```python
from build123d import *

# Parameters (mm, degrees)
BOSS_EXTRUDE1_DEPTH = 5
SKETCH2_W           = 20.5
SKETCH2_H           = 30
SKETCH2_R           = 3
SKETCH2_R_2         = 1.5
BOSS_EXTRUDE2_DEPTH = 5
FILLET1_R           = 10.25


with BuildPart() as part:
    # Sketch1 → Boss-Extrude1 (new body)
    with BuildSketch(Plane(origin=(0, 0, 0), x_dir=(1, 0, 0), z_dir=(0, 1, 0))):
        Polygon((44.375484097, 7.788988346), (75.375484097, 7.788988346), (80.375484097, 7.788988346), (80.375484097, 12.788988346), (75.375484097, 12.788988346), (75.375484097, 18.288988346), (73.375484097, 18.288988346), (73.375484097, 17.188988346), (71.075484097, 17.188988346), (71.075484097, 18.288988346), (68.375484097, 18.288988346), (68.375484097, 21.288988346), (71.075484097, 21.288988346), (71.075484097, 22.388988346), (73.375484097, 22.388988346), (73.375484097, 21.288988346), (75.375484097, 21.288988346), (75.375484097, 26.788988346), (80.375484097, 26.788988346), (80.375484097, 31.788988346), (75.375484097, 31.788988346), (44.375484097, 31.788988346), (39.375484097, 31.788988346), (39.375484097, 26.788988346), (44.375484097, 26.788988346), (44.375484097, 21.288988346), (46.375484097, 21.288988346), (46.375484097, 22.388988346), (48.675484097, 22.388988346), (48.675484097, 21.288988346), (51.375484097, 21.288988346), (51.375484097, 18.288988346), (48.675484097, 18.288988346), (48.675484097, 17.188988346), (46.375484097, 17.188988346), (46.375484097, 18.288988346), (44.375484097, 18.288988346), (44.375484097, 12.788988346), (39.375484097, 12.788988346), (39.375484097, 7.788988346), align=None)
    extrude(amount=BOSS_EXTRUDE1_DEPTH)

    # Sketch2 → Boss-Extrude2 (add)
    with BuildSketch(Plane(origin=(0, 5, 0), x_dir=(1, 0, 0), z_dir=(0, 1, 0))):
        with Locations((59.875484097, -7.211011654)):
            Rectangle(SKETCH2_W, SKETCH2_H)
        with Locations(Location((59.875484097, -11.961011654, 0), (0, 0, 270))):
            Circle(SKETCH2_R, mode=Mode.SUBTRACT)
        with Locations(Location((59.875484097, -19.461011654, 0), (0, 0, 270))):
            Circle(SKETCH2_R_2, mode=Mode.SUBTRACT)
        with Locations(Location((52.375484097, -11.961011654, 0), (0, 0, 90))):
            Circle(SKETCH2_R_2, mode=Mode.SUBTRACT)
        with Locations(Location((67.375484097, -11.961011654, 0), (0, 0, 90))):
            Circle(SKETCH2_R_2, mode=Mode.SUBTRACT)
        with Locations(Location((59.875484097, -4.461011654, 0), (0, 0, 270))):
            Circle(SKETCH2_R_2, mode=Mode.SUBTRACT)
    extrude(amount=-BOSS_EXTRUDE2_DEPTH)

    # Fillet1
    fillet1_edges = [part.edges().sort_by_distance(p)[0] for p in [
        (49.625484097, 2.5, 22.211011654),
        (70.125484097, 2.5, 22.211011654),
    ]]
    fillet(fillet1_edges, radius=FILLET1_R - 0.0001)  # a hair under: the kernel refuses the full size


solid = part.part
```
CAD build for the part. Positions are in the model's coordinates, mm. A direction names the side the tool comes from. Round coordinates to 2 decimals unless told otherwise and drop trailing zeros. Loops run counter-clockwise (first coordinate to the right, second up) from the corner with the lowest first, then second, coordinate; pieces in that order, holes last. Notation, with made-up numbers: M 2,83 L 22,83 A21 cw 22,117 Z; hole C 37,-29 d6. An arc over 180 degrees is marked long. Use a Markdown table: item, result. Add a question column.
(1) Cut at C-C (z = 1.5). Give the cut face in (x, y).
(2) Which spindle directions (+Z, -Z, +X, -X, +Y, -Y) get a long thin tool onto all of the face, cutting with end or side? Do faces 5 (the face through (39.375, 2, -10)), 6 (the face through (73.375, 2, -18)), 7 (the face through (75.375, 2, -16)), 8 (the face through (50, 2, -18.289)). Say none if no direction does.
(3) Drill centre lines: line 1 (Z direction, x = 46, y = 0.45); line 2 (Z direction, x = 76, y = 3.7); line 3 (Z direction, x = 51, y = 3.25). Where is each one in solid material? Low to high.
(4) Pull direction Z, two halves, no side cores. Call faces 1 (the face through (60, 2, -31.789)), 2 (the face through (45, 2, -21.289)), 3 (the face through (52.71, 2.46, 19.29)), 4 (the face through (42, 2, -26.789)): +Z half, -Z half, draft (parallel to the pull), parting line (faces both ways), or undercut.
(5) Cut at B-B (x = 77). Give the cut face in (y, z).
(6) Flat gauge pins, fed straight in: pin 1 (0.9 mm diameter, centred on y = 2, z = -22, fed in from +X); pin 2 (2.5 mm diameter, centred on x = 59.88, z = 4.46, fed in from +Y); pin 3 (0.9 mm diameter, centred on y = 2.5, z = -17.5, fed in from -X); pin 4 (1.2 mm diameter, centred on x = 48, y = 1.5, fed in from +Z). Where does each tip first touch, or does it go through?
(7) Cut at D-D (y = 3.5). State how many separate pieces and enclosed holes the cut face has, and give its area (3 significant figures).
(8) Cut at A-A (x = 72). Give the cut face in (y, z).
Geometry says:
| question | item | result |
|---|---|---|
| 1 | outline | M 49.63,0 L 70.13,0 L 70.13,5 L 49.63,5 Z |
| 2 | face 5 | +Z, -Z, -X, +Y, -Y |
| 2 | face 6 | +Y, -Y |
| 2 | face 7 | +X, +Y, -Y |
| 2 | face 8 | -X, +Y, -Y |
| 3 | line 1 | z = -31.79 to -21.29, -18.29 to -7.79 |
| 3 | line 2 | z = -31.79 to -26.79, -12.79 to -7.79 |
| 3 | line 3 | z = -31.79 to -21.29, -18.29 to 11.36, 12.56 to 17.09 |
| 4 | face 1 | -Z half |
| 4 | face 2 | undercut |
| 4 | face 3 | +Z half |
| 4 | face 4 | undercut |
| 5 | outline | M 0,-31.79 L 5,-31.79 L 5,-26.79 L 0,-26.79 Z; M 0,-12.79 L 5,-12.79 L 5,-7.79 L 0,-7.79 Z |
| 6 | pin 1 | stops at x = 75.38 |
| 6 | pin 2 | passes through |
| 6 | pin 3 | stops at x = 44.38 |
| 6 | pin 4 | stops at z = -7.79 |
| 7 | separate pieces | 1 |
| 7 | enclosed holes | 5 |
| 7 | area | 1,310 mm² |
| 8 | outline | M 0,-31.79 L 5,-31.79 L 5,-22.39 L 0,-22.39 Z; M 0,-17.19 L 5,-17.19 L 5,-7.79 L 0,-7.79 Z |
